```python
from build123d import *

# Parameters (mm, degrees)
BOSS_EXTRUDE1_DEPTH         = 6.35
SKETCH6_R                   = 25.4
CUT_EXTRUDE1_DEPTH          = 1658.310568825
F_1_4_0_25_DIAMETER_HOLE1_D = 6.35
CIRPATTERN1_COUNT           = 8


with BuildPart() as part:
    # Sketch5 → Boss-Extrude1 (new body)
    with BuildSketch(Plane(origin=(0, 0, 0), x_dir=(1, 0, 0), z_dir=(0, 1, 0))):
        with BuildLine():
            Line((-947.592639328, 61.760579697), (-1554.544647829, 30.079641))
            Line((-1554.544647829, 30.079641), (-1656.144647829, 30.079641))
            Line((-1656.144647829, 30.079641), (-1656.144647829, -8.020359))
            Line((-1656.144647829, -8.020359), (-1554.544647829, -8.020359))
            Line((-1554.544647829, -8.020359), (-947.592639328, -39.701297696))
            ThreePointArc((-947.592639328, -39.701297696), (-894.144647829, 11.029641), (-947.592639328, 61.760579697))
        make_face()
    extrude(amount=BOSS_EXTRUDE1_DEPTH)

    # Sketch6 → Cut-Extrude1 (cut, through all)
    with BuildSketch(Plane(origin=(0, 6.35, 0), x_dir=(1, 0, 0), z_dir=(0, 1, 0))):
        with Locations(Location((-944.944647829, 11.029641, 0), (0, 0, 270))):
            Circle(SKETCH6_R)
    extrude(amount=-CUT_EXTRUDE1_DEPTH, mode=Mode.SUBTRACT)

    # 1/4 (0.25) Diameter Hole1 (through all)
    with Locations(Plane(origin=(0, 6.35, 0), x_dir=(1, 0, 0), z_dir=(0, 1, 0))):
        with Locations((-944.944647829, 49.129641)):
            f_1_4_0_25_diameter_hole1 = Hole(F_1_4_0_25_DIAMETER_HOLE1_D / 2)

    # CirPattern1: 1/4 (0.25) Diameter Hole1 ×8 about axis
    cirpattern1_axis = Axis((-944.944647829, 0, -11.029641), (0, 1, 0))
    for i in range(1, CIRPATTERN1_COUNT):
        add(f_1_4_0_25_diameter_hole1.rotate(cirpattern1_axis, i * 360 / CIRPATTERN1_COUNT), mode=Mode.SUBTRACT)


solid = part.part
```
Here's how the part is built. I have some questions about the finished solid (model axes, mm). Coordinates: 2 decimals unless noted, no trailing zeros. Order: outer loops, then holes, each group sorted by start corner. A loop starts at its lowest first (then second) coordinate and runs counter-clockwise, first axis right, second up.
1) Imagine slicing it at D-D on x = -1393.5. List the corners of the cut face in (y, z) for me.
2) Imagine slicing it at A-A on z = 0.5. List the corners of the cut face in (x, y) for me, and give its area (3 significant figures).
3) Will these pins go through, and if not, where does the flat tip stop? pin 1 (2 mm diameter, centred on y = 3, z = 2.5, fed in from +X); pin 2 (1 mm diameter, centred on x = -973, y = 1, fed in from +Z); pin 3 (1 mm diameter, centred on x = -1568.5, y = 4, fed in from -Z).
4) We'd pull the mould along X, two halves only. Please class faces 1 (the face through (-1196, 6.35, -12)), 2 (the face through (-969.74, 3.22, -16.54)), 3 (the face through (-1246.82, 3.13, -46.14)): +X half, -X half, draft (parallel to the pull), parting line (faces both ways), or undercut.
5) Imagine slicing it at C-C on x = -1096.5. List the corners of the cut face in (y, z) for me.
6) Imagine slicing it at B-B on y = 4.75. State how many separate pieces and enclosed holes the cut face has, and give its area (3 significant figures).
7) I need wall thicknesses on line 1 (X direction, y = 5.75, z = -8.5); line 2 (X direction, y = 2.75, z = -4); line 3 (X direction, y = 6, z = 6.5). Which ranges of each line are inside material? Lowest first, please.
Response values:
1. outline: (0, -38.49) - (6.35, -38.49) - (6.35, 16.43) - (0, 16.43) - close
2. outline: (-1656.14, 0) - (-967.58, 0) - (-967.58, 6.35) - (-1656.14, 6.35) - close; (-922.31, 0) - (-895.47, 0) - (-895.47, 6.35) - (-922.31, 6.35) - close
2. area: 4,540 mm2
3. pin 1: stops at x = -895.71
3. pin 2: stops at z = 38.4
3. pin 3: stops at z = -30.08
4. face 1: draft
4. face 2: undercut
4. face 3: -X half
5. outline: (0, -53.99) - (6.35, -53.99) - (6.35, 31.93) - (0, 31.93) - close
6. separate pieces: 1
6. enclosed holes: 9
6. area: 48,300 mm2
7. line 1: x = -1656.14 to -984.96, -981.13 to -970.22, -919.67 to -908.76, -904.93 to -894.21
7. line 2: x = -1656.14 to -969.35, -920.54 to -894.63
7. line 3: x = -1656.14 to -963.33, -926.56 to -897.26
